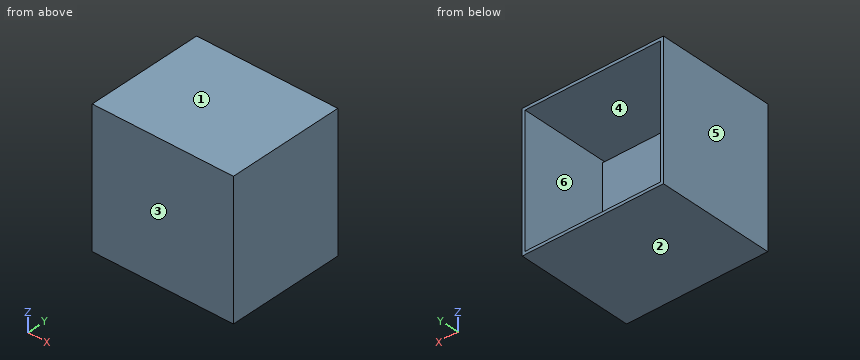
```python
from build123d import *

# Parameters (mm, degrees)
F0_W      = 70
F0_H      = 40
F1_DEPTH  = 25
F2_DEPTH  = 25
F3_DEPTH  = 25
F4_DEPTH  = 25
F5_DEPTH  = 25
F6_DEPTH  = 25
F7_DEPTH  = 25
F8_DEPTH  = 25
F9_DEPTH  = 25
F10_T     = -2.5
F11_W     = 111.0436096787
F11_H     = 98.0712249875
F12_DEPTH = 25


with BuildPart() as f1:
    # F0 (on Front) → F1 (new body)
    with BuildSketch(Plane.XZ):
        with Locations((-3.5461261868, 0)):
            Rectangle(F0_W, F0_H)
    extrude(amount=F1_DEPTH)

    # F2 (add): a face of the model
    f2_faces = [f1.faces().sort_by_distance(p)[0] for p in [
        (-38.5461261868, -12.5, 0),
    ]]
    extrude(f2_faces, amount=F2_DEPTH)

    # F3 (add): a face of the model
    f3_faces = [f1.faces().sort_by_distance(p)[0] for p in [
        (-63.5461261868, -12.5, 0),
    ]]
    extrude(f3_faces, amount=F3_DEPTH)

    # F4 (add): a face of the model
    f4_faces = [f1.faces().sort_by_distance(p)[0] for p in [
        (-28.5461261868, -12.5, 20),
    ]]
    extrude(f4_faces, amount=F4_DEPTH)

    # F5 (add): a face of the model
    f5_faces = [f1.faces().sort_by_distance(p)[0] for p in [
        (-28.5461261868, -12.5, 45),
    ]]
    extrude(f5_faces, amount=F5_DEPTH)

    # F6 (add): a face of the model
    f6_faces = [f1.faces().sort_by_distance(p)[0] for p in [
        (-28.5461261868, -25, 25),
    ]]
    extrude(f6_faces, amount=F6_DEPTH)

    # F7 (add): a face of the model
    f7_faces = [f1.faces().sort_by_distance(p)[0] for p in [
        (-28.5461261868, -50, 25),
    ]]
    extrude(f7_faces, amount=F7_DEPTH)

    # F8 (add): a face of the model
    f8_faces = [f1.faces().sort_by_distance(p)[0] for p in [
        (-28.5461261868, 0, 25),
    ]]
    extrude(f8_faces, amount=F8_DEPTH)

    # F9 (add): a face of the model
    f9_faces = [f1.faces().sort_by_distance(p)[0] for p in [
        (-28.5461261868, -25, 70),
    ]]
    extrude(f9_faces, amount=F9_DEPTH)

    # F10
    f10_openings = [f1.faces().sort_by_distance(p)[0] for p in [
        (-28.546126, 25, 37.5),
    ]]
    offset(amount=F10_T, openings=f10_openings)

    # F11 (on face) → F12 (join)
    with BuildSketch(Plane(origin=(0, -72.5, 0), x_dir=(-1, 0, 0), z_dir=(0, 1, 0))):
        with Locations((27.7883224189, 40.0959290564)):
            Rectangle(F11_W, F11_H)
    extrude(amount=F12_DEPTH)


solid = f1.part
```
Could you check a few things on this model? Use its own coordinates, in mm. Face numbers are marked on the shaded views. A direction names the side the tool comes from. Give positions to 0.01 mm unless a question says otherwise; leave off trailing zeros. Order: outer loops, then holes, each group sorted by start corner. A loop starts at its lowest first (then second) coordinate and runs counter-clockwise, first axis right, second up.
Q1. Suppose I cut it at A-A, the plane y = -50.5. Write out the boundary of the cut face in (x, z).
Q2. I'm going to push a flat-ended pin straight in: P1, Ø1, axis at x = -2.5, z = 57, coming from the +Y side. Where does the tip first touch, or does it pass through?
Q3. Suppose I cut it at D-D, the plane y = -22.5. Write out the boundary of the cut face in (x, z), and give its area (3 significant figures).
Q4. Suppose I cut it at C-C, the plane x = -20. Write out the boundary of the cut face in (y, z).
Q5. We'd pull the mould along Z, two halves only. Please class the marked faces 1, 2, 3 and 4: +Z half, -Z half, draft (parallel to the pull), parting line (faces both ways), or undercut.
Q6. If I drill on line 1 along Z through (x, y) = (-79, -54); line 2 along X through (y, z) = (-51, 64); line 3 along Z through (x, y) = (-32, -31), over which ranges is the centre line in solid material (lowest first)?
Q7. For the marked faces 5 and 6, which set-ups out of +Z, -Z, +X, -X, +Y, -Y let a thin tool reach every point of the face, with its end or its side?
Q8. Suppose I cut it at B-B, the plane z = 2.5. Write out the boundary of the cut face in (x, y).
Solution:
1. outline: (-88.55, -20) - (31.45, -20) - (31.45, 95) - (-88.55, 95) - close; (-83.31, -8.94) - (27.73, -8.94) - (27.73, 89.13) - (-83.31, 89.13) - close; hole (-86.05, -17.5) - (28.95, -17.5) - (28.95, 92.5) - (-86.05, 92.5) - close
2. P1: stops at y = -47.5
3. outline: (-88.55, -20) - (31.45, -20) - (31.45, 95) - (-88.55, 95) - close; hole (-86.05, -17.5) - (28.95, -17.5) - (28.95, 92.5) - (-86.05, 92.5) - close
3. area: 1,150 mm2
4. outline: (-75, -20) - (25, -20) - (25, -17.5) - (-72.5, -17.5) - (-72.5, -8.94) - (-47.5, -8.94) - (-47.5, 89.13) - (-72.5, 89.13) - (-72.5, 92.5) - (25, 92.5) - (25, 95) - (-75, 95) - close
5. face 1: +Z half
5. face 2: -Z half
5. face 3: draft
5. face 4: undercut
6. line 1: z = -20 to -17.5, -8.94 to 89.13, 92.5 to 95
6. line 2: x = -88.55 to -86.05, -83.31 to 27.73, 28.95 to 31.45
6. line 3: z = -20 to -17.5, 92.5 to 95
7. face 5: +Z, -Z, -X, +Y, -Y
7. face 6: +Y
8. outline: (-88.55, -75) - (31.45, -75) - (31.45, 25) - (28.95, 25) - (28.95, -72.5) - (27.73, -72.5) - (27.73, -47.5) - (-83.31, -47.5) - (-83.31, -72.5) - (-86.05, -72.5) - (-86.05, 25) - (-88.55, 25) - close
